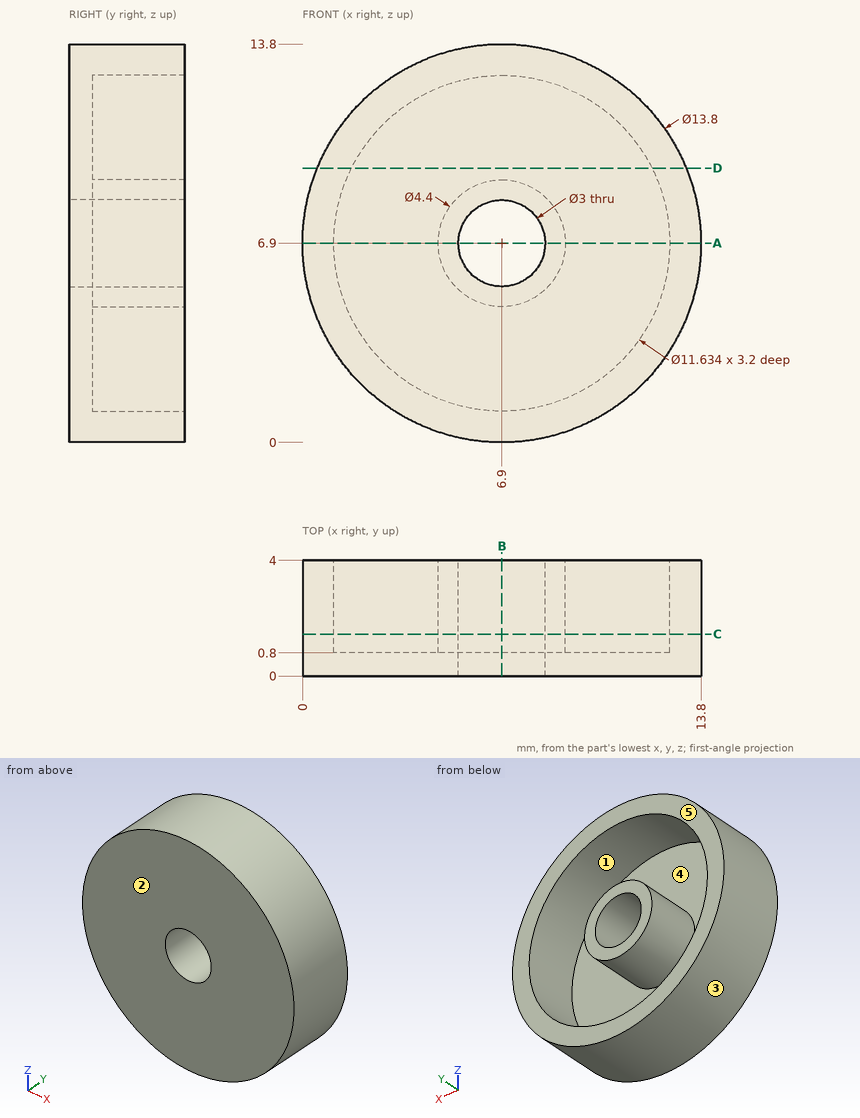
Could you check a few things on this drawing? It's one solid part, dimensions in mm from its lowest x, y, z. A direction names the side the tool comes from. Round coordinates to 2 decimals unless told otherwise and drop trailing zeros. Loops run counter-clockwise (first coordinate to the right, second up) from the corner with the lowest first, then second, coordinate; pieces in that order, holes last. Notation, with made-up numbers: (-11.5, 39) -> (42.5, 39) arc R16 ccw to (42.5, 61) -> close; hole circle Ø11 at (87.25, 19.25). An arc over 180 degrees is marked (long way). One line per item, written item: value. Start each with the question number.
1. For pin 1 (1.5 mm diameter, centred on x = 9, z = 10.5, fed in from +Y); pin 2 (1.5 mm diameter, centred on x = 9.5, y = 1.5, fed in from +Z); pin 3 (2 mm diameter, centred on y = 3, z = 10, fed in from -X), each with a flat end and sliding along its axis, tell me the tip position at first contact or that it passes through.
2. If I drill on probe 1 along X at (y, z) = (2.9, 6.9); probe 2 along X at (y, z) = (3.1, 7.75) (1 decimal); probe 3 along X at (y, z) = (3.4, 5) (1 decimal), over which ranges is the centre line in solid material (lowest first)?
3. If we section it at D-D, the plane z = 9.5: Write out the boundary of the cut face in (x, y), then the cut area to 3 significant figures.
4. If we section it at B-B, the plane x = 6.9: Write out the boundary of the cut face in (y, z).
5. If we section it at C-C, the plane y = 1.45: Write out the boundary of the cut face in (x, z).
6. If we section it at A-A, the plane z = 6.9: Write out the boundary of the cut face in (x, y).
7. If we mould it in two halves opening along Z, with no side actions, what happens to the marked faces 1, 2 and 3? For each: pulls with the +Z half, pulls with the -Z half, needs draft (parallel to the pull), parting line crosses it, or undercut.
8. For the marked faces 4 and 5, which set-ups out of +Z, -Z, +X, -X, +Y, -Y let a thin tool reach every point of the face, with its end or its side?
Calculated:
1. pin 1: stops at y = 0.8
1. pin 2: stops at z = 13.55
1. pin 3: stops at x = 0.33
2. probe 1: x = 0 to 1.08, 4.7 to 5.4, 8.4 to 9.1, 12.72 to 13.8
2. probe 2: x = 0.1 to 1.1, 4.9 to 5.7, 8.1 to 8.9, 12.7 to 13.7
2. probe 3: x = 0.3 to 1.4, 5.8 to 8, 12.4 to 13.5
3. outline: (0.51, 0) -> (13.29, 0) -> (13.29, 4) -> (12.1, 4) -> (12.1, 0.8) -> (1.7, 0.8) -> (1.7, 4) -> (0.51, 4) -> close
3. area: 17.8 mm²
4. outline: (0, 0) -> (4, 0) -> (4, 1.08) -> (0.8, 1.08) -> (0.8, 4.7) -> (4, 4.7) -> (4, 5.4) -> (0, 5.4) -> close; (0, 8.4) -> (4, 8.4) -> (4, 9.1) -> (0.8, 9.1) -> (0.8, 12.72) -> (4, 12.72) -> (4, 13.8) -> (0, 13.8) -> close
5. outline: circle Ø13.8 at (6.9, 6.9); circle Ø4.4 at (6.9, 6.9); hole circle Ø11.63 at (6.9, 6.9); hole circle Ø3 at (6.9, 6.9)
6. outline: (0, 0) -> (5.4, 0) -> (5.4, 4) -> (4.7, 4) -> (4.7, 0.8) -> (1.08, 0.8) -> (1.08, 4) -> (0, 4) -> close; (8.4, 0) -> (13.8, 0) -> (13.8, 4) -> (12.72, 4) -> (12.72, 0.8) -> (9.1, 0.8) -> (9.1, 4) -> (8.4, 4) -> close
7. face 1: undercut
7. face 2: needs draft
7. face 3: parting line crosses it
8. face 4: +Y
8. face 5: +Z, -Z, +X, -X, +Y
